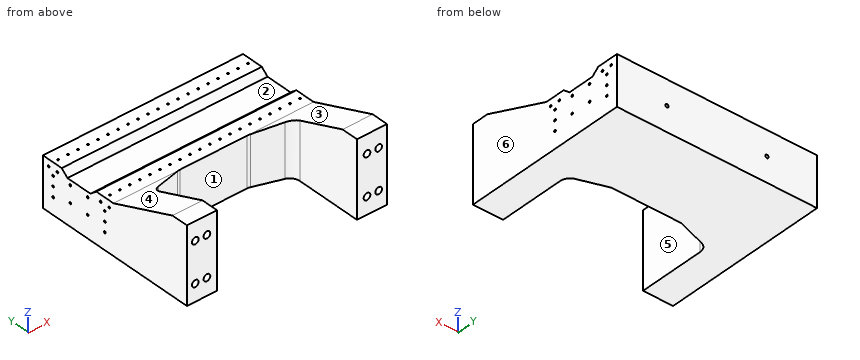
```python
from build123d import *

# Parameters (mm, degrees)
SKETCH1_W                  = 600
SKETCH1_H                  = 500
BOSS_EXTRUDE1_DEPTH        = 226
SKETCH2_OUTSIDE_W          = 764.614
SKETCH2_OUTSIDE_H          = 664.614
CUT_EXTRUDE1_DEPTH         = 452.193971591
CUT_EXTRUDE8_DEPTH         = 452.193971591
CUT_EXTRUDE2_DEPTH         = 689.168583997
CUT_EXTRUDE3_DEPTH         = 689.168583997
SKETCH7_R                  = 2.5
CUT_EXTRUDE5_DEPTH         = 25
SKETCH8_R                  = 10
CUT_EXTRUDE6_DEPTH         = 35
F_6_0MM_DOWEL_HOLE1_D      = 6
F_6_0MM_DOWEL_HOLE1_DEPTH  = 28.197418143
F_6_0MM_DOWEL_HOLE1_TIP    = 1.802581857
F_6_0MM_DOWEL_HOLE2_D      = 6
F_6_0MM_DOWEL_HOLE2_DEPTH  = 28.197418143
F_6_0MM_DOWEL_HOLE2_TIP    = 1.802581857
F_6_0MM_DOWEL_HOLE3_D      = 6
F_6_0MM_DOWEL_HOLE3_DEPTH  = 28.197418143
F_6_0MM_DOWEL_HOLE3_TIP    = 1.802581857
FILLET2_R                  = 30
F_6_0MM_DOWEL_HOLE4_D      = 6
F_6_0MM_DOWEL_HOLE4_DEPTH  = 28
F_6_0MM_DOWEL_HOLE4_TIP    = 1.802581857
F_10_0MM_DOWEL_HOLE1_D     = 10
F_10_0MM_DOWEL_HOLE1_DEPTH = 28
F_10_0MM_DOWEL_HOLE1_TIP   = 3.004303095


with BuildPart() as part:
    # Sketch1 → Boss-Extrude1 (new body)
    with BuildSketch(Plane.XY):
        Rectangle(SKETCH1_W, SKETCH1_H)
    extrude(amount=BOSS_EXTRUDE1_DEPTH)

    # Sketch2 outside → Cut-Extrude1 (cut, through all)
    with BuildSketch(Plane.XY.offset(226)):
        Rectangle(SKETCH2_OUTSIDE_W, SKETCH2_OUTSIDE_H)
        Polygon((-210, -250), (-210, -225), (-210, -30), (210, -30), (210, -225), (210, -250), (300, -250), (300, 250), (-300, 250), (-300, -250), align=None, mode=Mode.SUBTRACT)
    extrude(amount=-CUT_EXTRUDE1_DEPTH, mode=Mode.SUBTRACT)

    # Sketch22 → Cut-Extrude8 (cut, through all)
    with BuildSketch(Plane.XY.offset(226)):
        Polygon((-210, -30), (210, -30), (105, 5), (0, 5), (-105, 5), align=None)
    extrude(amount=-CUT_EXTRUDE8_DEPTH, mode=Mode.SUBTRACT)

    # Sketch4 → Cut-Extrude2 (cut, through all)
    with BuildSketch(Plane.ZY.offset(300)):
        Polygon((148, 25), (148, 5), (226, -200), (226, -165), (226, -145), (226, 250), (148, 250), align=None)
    extrude(amount=-CUT_EXTRUDE2_DEPTH, mode=Mode.SUBTRACT)

    # Sketch5 → Cut-Extrude3 (cut, through all)
    with BuildSketch(Plane.ZY.offset(300)):
        Polygon((131, 160), (131, 165), (148, 185), (148, 65), (131, 85), (131, 90), (131, 125), align=None)
    extrude(amount=-CUT_EXTRUDE3_DEPTH, mode=Mode.SUBTRACT)

    # Sketch7 → Cut-Extrude5 (cut)
    with BuildSketch(Plane.XY.offset(148)):
        with Locations((-285, 215)):
            Circle(SKETCH7_R)
        with Locations((-255, 215)):
            Circle(SKETCH7_R)
        with Locations((-225, 215)):
            Circle(SKETCH7_R)
        with Locations((-195, 215)):
            Circle(SKETCH7_R)
        with Locations((-165, 215)):
            Circle(SKETCH7_R)
        with Locations((-135, 215)):
            Circle(SKETCH7_R)
        with Locations((-105, 215)):
            Circle(SKETCH7_R)
        with Locations((-75, 215)):
            Circle(SKETCH7_R)
        with Locations((-45, 215)):
            Circle(SKETCH7_R)
        with Locations((-15, 215)):
            Circle(SKETCH7_R)
        with Locations((15, 215)):
            Circle(SKETCH7_R)
        with Locations((45, 215)):
            Circle(SKETCH7_R)
        with Locations((75, 215)):
            Circle(SKETCH7_R)
        with Locations((105, 215)):
            Circle(SKETCH7_R)
        with Locations((135, 215)):
            Circle(SKETCH7_R)
        with Locations((165, 215)):
            Circle(SKETCH7_R)
        with Locations((195, 215)):
            Circle(SKETCH7_R)
        with Locations((225, 215)):
            Circle(SKETCH7_R)
        with Locations((255, 215)):
            Circle(SKETCH7_R)
        with Locations((285, 215)):
            Circle(SKETCH7_R)
        with Locations((-255, 35)):
            Circle(SKETCH7_R)
        with Locations((-225, 35)):
            Circle(SKETCH7_R)
        with Locations((-195, 35)):
            Circle(SKETCH7_R)
        with Locations((-165, 35)):
            Circle(SKETCH7_R)
        with Locations((-135, 35)):
            Circle(SKETCH7_R)
        with Locations((-105, 35)):
            Circle(SKETCH7_R)
        with Locations((-75, 35)):
            Circle(SKETCH7_R)
        with Locations((-45, 35)):
            Circle(SKETCH7_R)
        with Locations((-15, 35)):
            Circle(SKETCH7_R)
        with Locations((15, 35)):
            Circle(SKETCH7_R)
        with Locations((45, 35)):
            Circle(SKETCH7_R)
        with Locations((75, 35)):
            Circle(SKETCH7_R)
        with Locations((105, 35)):
            Circle(SKETCH7_R)
        with Locations((135, 35)):
            Circle(SKETCH7_R)
        with Locations((165, 35)):
            Circle(SKETCH7_R)
        with Locations((195, 35)):
            Circle(SKETCH7_R)
        with Locations((225, 35)):
            Circle(SKETCH7_R)
        with Locations((255, 35)):
            Circle(SKETCH7_R)
        with Locations((285, 35)):
            Circle(SKETCH7_R)
        with Locations((-285, 35)):
            Circle(SKETCH7_R)
    extrude(amount=-CUT_EXTRUDE5_DEPTH, mode=Mode.SUBTRACT)

    # Sketch8 → Cut-Extrude6 (cut)
    with BuildSketch(Plane.XZ.offset(250)):
        with Locations((240, 171)):
            Circle(SKETCH8_R)
        with Locations((275, 171)):
            Circle(SKETCH8_R)
        with Locations((240, 51)):
            Circle(SKETCH8_R)
        with Locations((275, 51)):
            Circle(SKETCH8_R)
        with Locations((-275, 51)):
            Circle(SKETCH8_R)
        with Locations((-240, 51)):
            Circle(SKETCH8_R)
        with Locations((-275, 171)):
            Circle(SKETCH8_R)
        with Locations((-240, 171)):
            Circle(SKETCH8_R)
    extrude(amount=-CUT_EXTRUDE6_DEPTH, mode=Mode.SUBTRACT)

    # Ø6.0mm Dowel Hole1
    with Locations(Plane.ZY.offset(300)):
        with Locations((116, 95), (66, 95), (66, 155), (116, 155), (128, 230), (128, 200), (128, 50), (128, 20)):
            Hole(F_6_0MM_DOWEL_HOLE1_D / 2, depth=F_6_0MM_DOWEL_HOLE1_DEPTH)
            with Locations((0, 0, -(F_6_0MM_DOWEL_HOLE1_DEPTH + F_6_0MM_DOWEL_HOLE1_TIP / 2))):  # 118° drill point
                Cone(0, F_6_0MM_DOWEL_HOLE1_D / 2, F_6_0MM_DOWEL_HOLE1_TIP, mode=Mode.SUBTRACT)

    # Ø6.0mm Dowel Hole2
    with Locations(Plane(origin=(300, 0, 0), x_dir=(0, 0, -1), z_dir=(1, 0, 0))):
        with Locations((-128, 230), (-128, 200), (-116, 155), (-66, 155), (-66, 95), (-116, 95), (-128, 50), (-128, 20)):
            Hole(F_6_0MM_DOWEL_HOLE2_D / 2, depth=F_6_0MM_DOWEL_HOLE2_DEPTH)
            with Locations((0, 0, -(F_6_0MM_DOWEL_HOLE2_DEPTH + F_6_0MM_DOWEL_HOLE2_TIP / 2))):  # 118° drill point
                Cone(0, F_6_0MM_DOWEL_HOLE2_D / 2, F_6_0MM_DOWEL_HOLE2_TIP, mode=Mode.SUBTRACT)

    # Ø6.0mm Dowel Hole3
    with Locations(Plane(origin=(300, 0, 0), x_dir=(0, 0, -1), z_dir=(1, 0, 0))):
        with Locations((-110, 215), (-80, 215), (-50, 215), (-50, 35), (-80, 35), (-110, 35)):
            Hole(F_6_0MM_DOWEL_HOLE3_D / 2, depth=F_6_0MM_DOWEL_HOLE3_DEPTH)
            with Locations((0, 0, -(F_6_0MM_DOWEL_HOLE3_DEPTH + F_6_0MM_DOWEL_HOLE3_TIP / 2))):  # 118° drill point
                Cone(0, F_6_0MM_DOWEL_HOLE3_D / 2, F_6_0MM_DOWEL_HOLE3_TIP, mode=Mode.SUBTRACT)

    # Fillet2
    fillet2_edges = [part.edges().sort_by_distance(p)[0] for p in [
        (210, -30, 80.658536585),
        (-210, -30, 80.658536585),
        (-105, 5, 74),
        (105, 5, 74),
    ]]
    fillet(fillet2_edges, radius=FILLET2_R)

    # Ø6.0mm Dowel Hole4
    with Locations(Plane.ZY.offset(300)):
        with Locations((110, 215), (80, 215), (50, 215), (110, 35), (80, 35), (50, 35)):
            Hole(F_6_0MM_DOWEL_HOLE4_D / 2, depth=F_6_0MM_DOWEL_HOLE4_DEPTH)
            with Locations((0, 0, -(F_6_0MM_DOWEL_HOLE4_DEPTH + F_6_0MM_DOWEL_HOLE4_TIP / 2))):  # 118° drill point
                Cone(0, F_6_0MM_DOWEL_HOLE4_D / 2, F_6_0MM_DOWEL_HOLE4_TIP, mode=Mode.SUBTRACT)

    # Ø10.0mm Dowel Hole1
    with Locations(Plane(origin=(0, 250, 0), x_dir=(1, 0, 0), z_dir=(0, 1, 0))):
        with Locations((-150, -74), (150, -74)):
            Hole(F_10_0MM_DOWEL_HOLE1_D / 2, depth=F_10_0MM_DOWEL_HOLE1_DEPTH)
            with Locations((0, 0, -(F_10_0MM_DOWEL_HOLE1_DEPTH + F_10_0MM_DOWEL_HOLE1_TIP / 2))):  # 118° drill point
                Cone(0, F_10_0MM_DOWEL_HOLE1_D / 2, F_10_0MM_DOWEL_HOLE1_TIP, mode=Mode.SUBTRACT)


solid = part.part
```
The model under review builds one solid part; all positions refer to its coordinate system, in mm. Face numbers are marked on the shaded views. A direction names the side the tool comes from. Round coordinates to 2 decimals unless told otherwise and drop trailing zeros. Loops run counter-clockwise (first coordinate to the right, second up) from the corner with the lowest first, then second, coordinate; pieces in that order, holes last.
Item 1: For the marked faces 1, 2 and 3, list the 3-axis set-ups (+Z, -Z, +X, -X, +Y, -Y) from which the entire face can be reached by the end or side of a thin tool; tool diameter is ignored.
Determined:
face 1: +Z, -Z, -Y
face 2: +Z, +X, -X
face 3: +Z, +X, -X, +Y
Item 2: Clearance check with flat-ended pins moving along their axes: pin 1 Ø8 at (x, y) = (255, 215) entering from +Z; pin 2 Ø5 at (y, z) = (200, 128) entering from +X; pin 3 Ø12 at (x, z) = (-240, 51) entering from -Y. State where each tip first meets the part, or that it passes through.
Determined:
pin 1: stops at z = 148
pin 2: stops at x = 271.5
pin 3: stops at y = -215
Item 3: Take a section at A-A (y = -37). Write out the cut boundary in (x, z).
Determined:
outline: (-300, 0) - (-206.19, 0) - (-206.19, 163.98) - (-300, 163.98) - close; (206.19, 0) - (300, 0) - (300, 163.98) - (206.19, 163.98) - close
Item 4: Take a section at B-B (y = 177). Write out the cut boundary in (x, z).
Determined:
outline: (-300, 0) - (300, 0) - (300, 141.2) - (-300, 141.2) - close
Item 5: For line 1 (Y direction, x = 293, z = 80); line 2 (Z direction, x = -275, y = -222.5); line 3 (Z direction, x = -286.5, y = 35), list the stretches that pass through material, from the lowest coordinate up.
Determined:
line 1: y = -250 to 32, 38 to 212, 218 to 250
line 2: z = 0 to 41, 61 to 161, 181 to 226
line 3: z = 0 to 47, 53 to 77, 83 to 107, 113 to 123
Item 6: Mouldability with a two-part tool opening along X and no side actions: class the marked faces 4, 5 and 6 as released by +X, released by -X, zero draft, split by the parting line, or undercut.
Determined:
face 4: zero draft
face 5: undercut
face 6: released by +X
